```python
from build123d import *

# Parameters (mm, degrees)
F0_W           = 48
F0_H           = 63.5
F1_DEPTH       = 6
F2_R           = 5
F3_D           = 5
F4_D           = 6
F4_CSINK_D     = 12
F4_CSINK_ANGLE = 90


# Not quite as in the source:
# - a feature names something its author has since deleted; it is built from what else it names


with BuildPart() as f1:
    # F0 (on Top) → F1 (new body)
    with BuildSketch(Plane.XY):
        with Locations((0, 12.75)):
            Rectangle(F0_W, F0_H)
    extrude(amount=-F1_DEPTH)

    # F2
    f2_edges = [f1.edges().sort_by_distance(p)[0] for p in [
        (-24, -19, -3),
        (-24, 44.5, -3),
        (24, -19, -3),
        (24, 44.5, -3),
    ]]
    fillet(f2_edges, radius=F2_R)

    # F3 (through all)
    with Locations(Plane.XY):
        with Locations((16.5, 1), (-16.5, 1), (16.5, 37), (-16.5, 37)):
            Hole(F3_D / 2)

    # F4 (through all)
    with Locations(Plane.XY):
        with Locations((15, -9), (-15, -9)):
            CounterSinkHole(F4_D / 2, F4_CSINK_D / 2, counter_sink_angle=F4_CSINK_ANGLE)


solid = f1.part
```
Geometry: final body of the model. Coordinates: model frame, mm. Round coordinates to 2 decimals unless told otherwise and drop trailing zeros. Order: outer loops, then holes, each group sorted by start corner. A loop starts at its lowest first (then second) coordinate and runs counter-clockwise, first axis right, second up. Notation, with made-up numbers: (67.25, 0.5) -> (114.25, 0.5) arc R31 cw to (114.25, 32.5) -> close; hole circle Ø8 at (49, -2.75). An arc over 180 degrees is marked (long way). Write each question's results on one line, items separated by ' | '.
Q1. Ray query, line 1 along X through (y, z) = (-9, -3.8); line 2 along X through (y, z) = (2.5, -4.5); line 3 along Y through (x, z) = (-16.5, -2.5). Return the intervals inside material, ascending.
Response values:
line 1: -24 to -18, -12 to 12, 18 to 24 | line 2: -24 to -18.5, -14.5 to 14.5, 18.5 to 24 | line 3: -19 to -12.16, -5.84 to -1.5, 3.5 to 34.5, 39.5 to 44.5
Q2. Section query B-B (x = 15). Output: boundary loops of the cut face in (y, z).
Response values:
outline: (-19, -6) -> (-12, -6) -> (-12, -3) -> (-15, 0) -> (-19, 0) -> close; (-6, -6) -> (-1, -6) -> (-1, 0) -> (-3, 0) -> (-6, -3) -> close; (3, -6) -> (35, -6) -> (35, 0) -> (3, 0) -> close; (39, -6) -> (44.5, -6) -> (44.5, 0) -> (39, 0) -> close
Q3. Section query C-C (z = -1.75). Output: boundary loops of the cut face in (x, y).
Response values:
outline: (-24, -14) arc R5 ccw to (-19, -19) -> (19, -19) arc R5 ccw to (24, -14) -> (24, 39.5) arc R5 ccw to (19, 44.5) -> (-19, 44.5) arc R5 ccw to (-24, 39.5) -> close; hole circle Ø8.5 at (-15, -9); hole circle Ø5 at (-16.5, 1); hole circle Ø5 at (-16.5, 37); hole circle Ø8.5 at (15, -9); hole circle Ø5 at (16.5, 1); hole circle Ø5 at (16.5, 37)
Q4. Pin query (flat end, axial travel): pin 1 Ø9.5 at (x, y) = (-15, -9) entering from +Z. Return the tip coordinate at first contact, or that it passes through.
Response values:
pin 1: z = -1.25
Q5. Section query A-A (y = 1). Output: boundary loops of the cut face in (x, z), and give its area (3 significant figures).
Response values:
outline: (-24, -6) -> (-19, -6) -> (-19, 0) -> (-24, 0) -> close; (-14, -6) -> (14, -6) -> (14, 0) -> (-14, 0) -> close; (19, -6) -> (24, -6) -> (24, 0) -> (19, 0) -> close | area: 228 mm²
Q6. Section query D-D (y = -9). Output: boundary loops of the cut face in (x, z), and give its area (3 significant figures).
Response values:
outline: (-24, -6) -> (-18, -6) -> (-18, -3) -> (-21, 0) -> (-24, 0) -> close; (-12, -6) -> (12, -6) -> (12, -3) -> (9, 0) -> (-9, 0) -> (-12, -3) -> close; (18, -6) -> (24, -6) -> (24, 0) -> (21, 0) -> (18, -3) -> close | area: 198 mm²
Q7. Pull-direction query (Y, two-part tool) for faces 1 (the face through (0, 13, -6)), 2 (the face through (22.57, 43, -3.04)), 3 (the face through (18, -9, -5)); classes: released by +Y, released by -Y, zero draft, split by the parting line, or undercut.
Response values:
face 1: zero draft | face 2: released by +Y | face 3: undercut
